Part model, mm, in its own coordinate system. Give positions to 0.01 mm unless a question says otherwise; leave off trailing zeros. Loops run counter-clockwise (first coordinate to the right, second up) from the corner with the lowest first, then second, coordinate; pieces in that order, holes last. Notation, with made-up numbers: (-18.5, 80.5) -> (13.5, 80.5) arc R17 ccw to (13.5, 91.5) -> close; hole circle Ø3 at (22.5, 30.5). An arc over 180 degrees is marked (long way). One line per question, with ' | ' between items.
Autodesk Inventor part; units mm, degrees
ref_plane "YZ Plane" through (0, 0, 0) normal (1, 0, 0) x (0, 1, 0)
ref_plane "XZ Plane" through (0, 0, 0) normal (0, 1, 0) x (-1, 0, 0)
ref_plane "XY Plane" through (0, 0, 0) normal (0, 0, 1) x (1, 0, 0)
sketch "Sketch1" plane through (0, 0, 0) normal (1, 0, 0) x (0, 1, 0)
  line L0 (0, 0) -> (-383, 0)
  line L1 (-383, 0) -> (-383, -1138)
  line L2 (-383, -1138) -> (0, -1138)
  line L3 (0, -1138) -> (0, 0)
  line L4 (-373, -1128) -> (-373, -10)
  line L5 (-373, -10) -> (-10, -10)
  line L6 (-10, -10) -> (-10, -1128)
  line L7 (-10, -1128) -> (-373, -1128)
  dimension "d0" = 383
  dimension "portaAltura" = 1138
  dimension "d2" = 10
  dimension "portaLargura" = 363
extrude "Extrusion1" add sketch "Sketch1" along normal blind 10
sketch "Sketch2" plane through (0, -383, 0) normal (0, 0, 1) x (1, 0, 0)
  line L0 (0, 383) -> (0, 0)
  line L1 (0, 0) -> (10, 0)
  line L2 (10, 383) -> (10, 0)
  line L3 (0, 383) -> (10, 383)
  line L4 (0, 0) -> (-3.182, -3.182)
  line L5 (0, 0) -> (4.5, 0) construction
  line L6 (0, 383) -> (0, 0)
  circle A0 centre (-3.182, -3.182) radius 5
  circle A1 centre (-3.182, -3.182) radius 4
  dimension "d5" = 4.5
  dimension "d6" = 135
  dimension "d7" = 1
  dimension "d10" = 10
extrude "Extrusion2" add sketch "Sketch2" against normal blind 35 contours A0 L1 L0 | L0 L1 A0
ref_plane "Work Plane1" through (0, 0, -569) normal (0, 0, 1) x (1, 0, 0)
mirror "Mirror1" about plane through (0, 0, -569) normal (0, 0, 1) of "Extrusion2"
fillet "Fillet1" [suppressed]
ref_plane "Work Plane2" through (0, -383, -1113) normal (0, 0, 1) x (1, 0, 0)
sketch "Sketch3" plane through (0, -383, -1113) normal (0, 0, 1) x (1, 0, 0)
  arc A0 (0, 0.6748) -> (0.6748, 0) centre (-3.182, -3.182) ccw
  circle A1 centre (-3.182, -3.182) radius 4
  line L0 (0.6748, 0) -> (10, 0)
  circle A2 centre (-3.182, -3.182) radius 5
  point P0 (0, 383)
  point P1 (0, 0.6748)
extrude "Extrusion3" cut sketch "Sketch3" against normal blind 15
sketch "Sketch4" plane through (0, 0, 0) normal (0, 0, 1) x (1, 0, 0)
  circle A0 centre (-3.182, -386.182) radius 4
  arc A1 (0, -382.3252) -> (0.6748, -383) centre (-3.182, -386.182) ccw
  circle A2 centre (-3.182, -386.182) radius 4
  line L0 (0.6748, -383) -> (10, -383)
  circle A3 centre (-3.182, -386.182) radius 5
  point P0 (0, 0)
  point P1 (0, -382.3252)
extrude "Extrusion4" cut sketch "Sketch4" against normal blind 10
sketch "Sketch5" plane through (0, -383, -35) normal (0, 0, -1) x (-1, 0, 0)
  circle A0 centre (3.182, -3.182) radius 4
  arc A1 (-0.6748, 0) -> (0, 0.6748) centre (3.182, -3.182) ccw
  circle A2 centre (3.182, -3.182) radius 5
  point P0 (0, 383)
  point P1 (0, 0.6748)
extrude "Extrusion5" cut sketch "Sketch5" against normal blind 10
sketch "Sketch6" plane through (0, 0, 0) normal (0, 0, 1) x (1, 0, 0)
  arc A0 (0.6748, -383) -> (0, -382.3252) centre (-3.182, -386.182) ccw
  line L0 (0.6748, -383) -> (10, -383)
  line L1 (10, 0) -> (10, -383)
  line L2 (0, 0) -> (10, 0)
  line L3 (0, 0) -> (0, -382.3252)
  line L4 (10, -383) -> (10, 0) construction
  line L5 (0, -10) -> (10, -10) construction
  line L6 (10, 0) -> (0, -10) construction
  line L7 (0, 0) -> (10, 0) construction
  line L8 (0, 0) -> (10, -10) construction
  circle A1 centre (5, -5) radius 2.5
  dimension "d19" = 5
extrude "Extrusion6" add sketch "Sketch6" along normal blind 10 contours A1
sketch "Sketch7" plane through (5, -5, 10) normal (0, 0, 1) x (1, 0, 0)
  circle A0 centre (0, 0) radius 2.5
  circle A1 centre (0, 0) radius 5
  point P0 (-5, 5)
  dimension "d22" = 10
extrude "Extrusion7" [suppressed]
mirror "Mirror2" about plane through (0, 0, -569) normal (0, 0, 1) of "Extrusion6"
properties part number "porta1"
1) Pin check, flat tips, straight feed: P1, Ø0.7, axis at x = 0.5, y = -382.5, coming from the +Z side; P2, Ø9, axis at x = -3.182, y = -386.182, coming from the +Z side; P3, Ø8, axis at x = 3.5, y = -208.5, coming from the -Z side. Stop position of each tip, or through.
Found:
P1: z = 0 | P2: z = -10 | P3: z = -1138
2) Saw through at C-C (x = -4.25). Give the cut face in (y, z), and give its area (3 significant figures).
Found:
outline: (-391.07, -1138) -> (-390.04, -1138) -> (-390.04, -1128) -> (-391.07, -1128) -> close; (-391.07, -1113) -> (-390.04, -1113) -> (-390.04, -1103) -> (-391.07, -1103) -> close; (-391.07, -25) -> (-390.04, -25) -> (-390.04, -10) -> (-391.07, -10) -> close; (-382.33, -1138) -> (-381.3, -1138) -> (-381.3, -1128) -> (-382.33, -1128) -> close; (-382.33, -1113) -> (-381.3, -1113) -> (-381.3, -1103) -> (-382.33, -1103) -> close; (-382.33, -25) -> (-381.3, -25) -> (-381.3, -10) -> (-382.33, -10) -> close | area: 72.1 mm2
3) Drill centre lines: line 1 (Y direction, x = 2, z = -173.5); line 2 (Z direction, x = 4.75, y = -314.5). Where is each one in solid material? Low to high.
Found:
line 1: -383 to -373, -10 to 0 | line 2: -1138 to -1128, -10 to 0
4) Saw through at A-A (z = -1018). Give the cut face in (x, y).
Found:
outline: (0, -383) -> (10, -383) -> (10, -373) -> (0, -373) -> close; (0, -10) -> (10, -10) -> (10, 0) -> (0, 0) -> close
5) Saw through at B-B (y = -160.5). Give the cut face in (x, z).
Found:
outline: (0, -1138) -> (10, -1138) -> (10, -1128) -> (0, -1128) -> close; (0, -10) -> (10, -10) -> (10, 0) -> (0, 0) -> close
